The listing builds one solid part. Answer for the finished solid, in the listing's coordinates (mm). Face numbers are marked on the shaded views. A direction names the side the tool comes from. Round coordinates to 2 decimals unless told otherwise and drop trailing zeros. Loops run counter-clockwise (first coordinate to the right, second up) from the corner with the lowest first, then second, coordinate; pieces in that order, holes last. Notation, with made-up numbers: (79, 7.25) -> (106, 7.25) arc R26 ccw to (106, 25.25) -> close; hole circle Ø5 at (66.25, 68.5). An arc over 180 degrees is marked (long way). Write each question's results on one line, items separated by ' | '. Start each with the question number.
(1) Determine the mould class of the marked faces 1, 2 and 3 for opening direction Z: released by +Z, released by -Z, zero draft, split by the parting line, or undercut.
(2) The part is cut by section A-A (y = 3). Determine the outline of the cut face in (x, z).
(3) The part is cut by section B-B (x = 28). Determine the outline of the cut face in (y, z), plus the area to 3 significant figures.
(4) For the marked faces 4, 5, 6 and 7, determine the directions among +Z, -Z, +X, -X, +Y, -Y from which every point of the face is accessible in a straight line to the end or side of a thin tool.
(5) Flat-ended cylindrical pins translate along their axes: pin 1 (12 mm diameter, centred on x = 41.5, y = 26.5, fed in from +Z); pin 2 (12 mm diameter, centred on y = 4.5, z = -12.5, fed in from -X); pin 3 (16.5 mm diameter, centred on y = 24.5, z = -22.5, fed in from +X). Find the tip coordinate at first contact, or state that the pin passes through.
(6) The part is cut by section D-D (x = 10). Determine the outline of the cut face in (y, z), plus the area to 3 significant figures.
(7) The part is cut by section C-C (z = -13.5). Determine the outline of the cut face in (x, y).
(8) Straight lines are drawn through the part: probe 1 along Z at (x, y) = (10, 32.5); probe 2 along Y at (x, z) = (16, -6.25); probe 3 along X at (y, z) = (27, -24.75). For each, find the intervals that lie inside material, in ascending order.
```python
from build123d import *

# Parameters (mm, degrees)
SKETCH1_W           = 70
SKETCH1_H           = 30
BOSS_EXTRUDE1_DEPTH = 35
CUT_EXTRUDE1_DEPTH  = 20
SKETCH3_W           = 20
SKETCH3_H           = 25
CUT_EXTRUDE2_DEPTH  = 31
SKETCH4_R           = 5
CUT_EXTRUDE3_DEPTH  = 36
SKETCH5_W           = 10
SKETCH5_H           = 5
CUT_EXTRUDE4_DEPTH  = 71


with BuildPart() as part:
    # Sketch1 → Boss-Extrude1 (new body)
    with BuildSketch(Plane(origin=(0, 0, 0), x_dir=(1, 0, 0), z_dir=(0, 1, 0))):
        with Locations((35, 15)):
            Rectangle(SKETCH1_W, SKETCH1_H)
    extrude(amount=BOSS_EXTRUDE1_DEPTH)

    # Sketch2 → Cut-Extrude1 (cut)
    with BuildSketch(Plane(origin=(0, 35, 0), x_dir=(1, 0, 0), z_dir=(0, 1, 0))):
        Polygon((70, 30), (50, 30), (50, 15), (35, 15), (35, 0), (70, 0), align=None)
    extrude(amount=-CUT_EXTRUDE1_DEPTH, mode=Mode.SUBTRACT)

    # Sketch3 → Cut-Extrude2 (cut, through all)
    with BuildSketch(Plane.XY):
        with Locations((10, 12.5)):
            Rectangle(SKETCH3_W, SKETCH3_H)
    extrude(amount=-CUT_EXTRUDE2_DEPTH, mode=Mode.SUBTRACT)

    # Sketch4 → Cut-Extrude3 (cut, through all)
    with BuildSketch(Plane(origin=(0, 35, 0), x_dir=(1, 0, 0), z_dir=(0, 1, 0))):
        with Locations((10, 15)):
            Circle(SKETCH4_R)
    extrude(amount=-CUT_EXTRUDE3_DEPTH, mode=Mode.SUBTRACT)

    # Sketch5 → Cut-Extrude4 (cut, through all)
    with BuildSketch(Plane(origin=(70, 0, 0), x_dir=(0, 0, -1), z_dir=(1, 0, 0))):
        with Locations((15, 2.5)):
            Rectangle(SKETCH5_W, SKETCH5_H)
    extrude(amount=-CUT_EXTRUDE4_DEPTH, mode=Mode.SUBTRACT)


solid = part.part
```
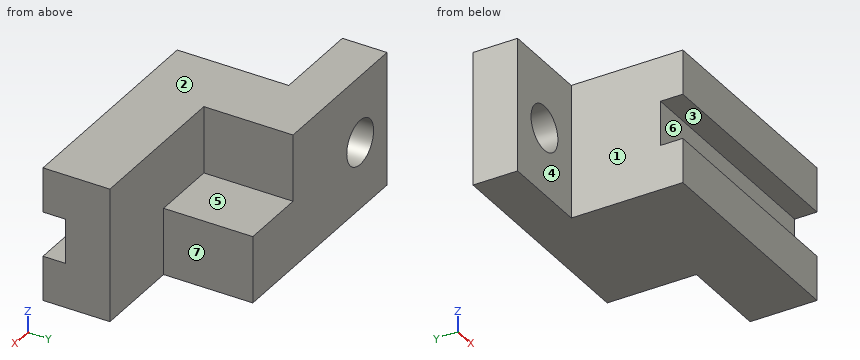
Checked values:
1) face 1: zero draft | face 2: released by +Z | face 3: undercut
2) outline: (20, -30) -> (70, -30) -> (70, -20) -> (20, -20) -> close; (20, -10) -> (70, -10) -> (70, 0) -> (20, 0) -> close
3) outline: (0, -30) -> (35, -30) -> (35, 0) -> (0, 0) -> (0, -10) -> (5, -10) -> (5, -20) -> (0, -20) -> close | area: 1,000 mm2
4) face 4: +Z, -Z, -X, -Y | face 5: +Z, +X, +Y | face 6: +X, -X, -Y | face 7: +Z, -Z, +X, +Y
5) pin 1: stops at z = -15 | pin 2: stops at x = 20 | pin 3: stops at x = 50
6) outline: (25, -30) -> (35, -30) -> (35, -20) -> (25, -20) -> close; (25, -10) -> (35, -10) -> (35, 0) -> (25, 0) -> close | area: 200 mm2
7) outline: (0, 25) -> (5.23, 25) -> (5.23, 35) -> (0, 35) -> close; (14.77, 25) -> (20, 25) -> (20, 5) -> (70, 5) -> (70, 15) -> (35, 15) -> (35, 35) -> (14.77, 35) -> close
8) probe 1: z = -30 to -20, -10 to 0 | probe 2: y = 25 to 35 | probe 3: x = 0 to 50
